```python
from build123d import *

# Parameters (mm, degrees)
BOSS_EXTRUDE1_DEPTH                 = 3.175
THICKNESS_REDUCTION_FOR_SIDES_DEPTH = 271.192313455


with BuildPart() as part:
    # Sketch2 → Boss-Extrude1 (new body)
    with BuildSketch(Plane.XY):
        with BuildLine():
            Line((-92.075, 0), (92.075, 0))
            Line((92.075, 0), (92.075, 236.855))
            ThreePointArc((92.075, 236.855), (87.053345763, 248.978345763), (74.93, 254))
            Line((74.93, 254), (-74.93, 254))
            ThreePointArc((-74.93, 254), (-87.053345763, 248.978345763), (-92.075, 236.855))
            Line((-92.075, 236.855), (-92.075, 0))
        make_face()
    extrude(amount=BOSS_EXTRUDE1_DEPTH)

    # Sketch4 → Thickness Reduction for sides (cut, through all)
    with BuildSketch(Plane.XY.offset(3.175)):
        with BuildLine():
            ThreePointArc((-74.93, 254), (-87.053345763, 248.978345763), (-92.075, 236.855))
            Line((-92.075, 236.855), (-92.075, 0))
            Line((-92.075, 0), (-88.9, 0))
            Line((-88.9, 0), (-88.9, 236.855))
            ThreePointArc((-88.9, 236.855), (-84.808281733, 246.733281733), (-74.93, 250.825))
            Line((-74.93, 250.825), (74.93, 250.825))
            ThreePointArc((74.93, 250.825), (84.808281733, 246.733281733), (88.9, 236.855))
            Line((88.9, 236.855), (88.9, 0))
            Line((88.9, 0), (92.075, 0))
            Line((92.075, 0), (92.075, 236.855))
            ThreePointArc((92.075, 236.855), (87.053345763, 248.978345763), (74.93, 254))
            Line((74.93, 254), (-74.93, 254))
        make_face()
    extrude(amount=-THICKNESS_REDUCTION_FOR_SIDES_DEPTH, mode=Mode.SUBTRACT)


solid = part.part
```
Can you work these out from the model? Positions are in its coordinate system, mm. Give positions to 0.01 mm unless a question says otherwise; leave off trailing zeros. Write item = value, one per line. Start each with the question number.
Q1. We'd pull the mould along Z, two halves only. Please class faces 1 (the cylindrical face through (84.7, 246.84, 1.61)), 2 (the flat face through (-1, 127, 0)), 3 (the flat face through (-1, 127, 3.175)): pulls with the +Z half, pulls with the -Z half, needs draft (parallel to the pull), parting line crosses it, or undercut.
Q2. Will this pin go through, and if not, where does the flat tip stop? pin 1 Ø5 at (x, y) = (1.5, 173) entering from -Z.
Q3. I need wall thicknesses on probe 1 along Y at (x, z) = (79, 2.8). Which ranges of the line are inside material? Lowest first, please. Write a range as [from, to].
Check result:
q1.face_1 = needs draft
q1.face_2 = pulls with the -Z half
q1.face_3 = pulls with the +Z half
q2.pin_1 = 0
q3.probe_1 = [0, 250.22]
